Read the model definition and answer for the solid it produces. Units are mm, in the model's axes. A direction names the side the tool comes from. Coordinates: 2 decimals unless noted, no trailing zeros. Order: outer loops, then holes, each group sorted by start corner. A loop starts at its lowest first (then second) coordinate and runs counter-clockwise, first axis right, second up. Notation, with made-up numbers: M 77,63.5 L 102,63.5 A17 cw 102,90.5 Z; hole C -24.5,-29.75 d7. An arc over 180 degrees is marked long. One line per question, with ' | ' between items. Start each with the question number.
1) Find section B-B, the plane z = 44.5. Write down the section's boundary in (x, y).
2) The mould has two halves that part along X. Classify faces 3 (the face through (-25, -1, 75)), 4 (the face through (-23.66, -0.67, 73.51)), 5 (the face through (-1, 50, 38)): +X half, -X half, draft (parallel to the pull), parting line (faces both ways), or undercut.
3) Consider probe 1 along Y at (x, z) = (-19, 58); probe 2 along Y at (x, z) = (-9, 16.5). Determine where each line is inside the solid, lowest interval first.
4) A tool of negligible diameter and unlimited length cuts with its end or side. For faces 1 (the face through (-1, -48, 48)), 2 (the face through (36.15, 0.36, 62.41)), from which of +Z, -Z, +X, -X, +Y, -Y can it reach the whole face along a straight path? Write none if from no direction.
5) Find section D-D, the plane z = 19. Write down the section's boundary in (x, y), plus the area to 3 significant figures.
6) Given P1, Ø1, axis at x = -2.5, y = -49.5, coming from the -Z side; P2, Ø10, axis at y = 39, z = 77.5, coming from the -X side; P3, Ø5, axis at x = 13.5, y = 39.5, coming from the -Z side, each flat-ended and moving along its own axis, determine where each tip first touches the part or whether it passes through.
from build123d import *

# Parameters (mm, degrees)
F0_W     = 100
F0_H     = 100
F1_DEPTH = 100
F2_SIZE2 = 49.99999
F2_SIZE  = 49.99999
F3_T     = -2
F4_W     = 23.5146284103
F4_H     = 39.5418182015
F5_DEPTH = 2
F7_D     = 12.6
F7_DEPTH = 17.25
F7_TIP   = 3.7854218999


# Not quite as in the source:
# - a fillet or chamfer is up to 0.001 mm smaller than in the source, because OpenCascade refuses the exact size


with BuildPart() as f1:
    # F0 (on Top) → F1 (new body)
    with BuildSketch(Plane.XY):
        Rectangle(F0_W, F0_H)
    extrude(amount=F1_DEPTH)

    # F2 (size 50 and 50 in the source; OpenCascade refuses exactly that, so slightly less here)
    f2_edges = [f1.edges().sort_by_distance(p)[0] for p in [
        (-50, 0, 100),
        (50, 0, 100),
    ]]
    chamfer(f2_edges, length=F2_SIZE, length2=F2_SIZE2)

    # F3
    f3_openings = [f1.faces().sort_by_distance(p)[0] for p in [
        (0, 0, 0),
    ]]
    offset(amount=F3_T, openings=f3_openings)

    # F4 (on face) → F5 (cut, through all)
    with BuildSketch(Plane.XZ.offset(50)):
        with Locations((-0.3359224647, 19.7709091008)):
            Rectangle(F4_W, F4_H)
    extrude(amount=-F5_DEPTH, mode=Mode.SUBTRACT)

    # F7
    with Locations(Plane(origin=(50, 0, 50), x_dir=(0, 1, 0), z_dir=(0.7071067812, 0, 0.7071067812))):
        with Locations((17.1098317951, 50.0659272075), (-10.7799200341, 50.0659272075), (-23.6778985709, 30.9631545097), (3.2679832075, 24.1581760347), (26.1959340423, 37.8756783903)):
            Hole(F7_D / 2, depth=F7_DEPTH)
            with Locations((0, 0, -(F7_DEPTH + F7_TIP / 2))):  # 118° drill point
                Cone(0, F7_D / 2, F7_TIP, mode=Mode.SUBTRACT)


solid = f1.part
Report:
1) outline: M -50,-50 L 50,-50 L 50,50 L -50,50 Z; hole M -48,-48 L 48,-48 L 48,48 L -48,48 Z
2) face 3: -X half | face 4: undercut | face 5: draft
3) probe 1: y = -50 to -48, 48 to 50 | probe 2: y = 48 to 50
4) face 1: -Z | face 2: none
5) outline: M -50,-50 L -12.09,-50 L -12.09,-48 L -48,-48 L -48,48 L 48,48 L 48,-48 L 11.42,-48 L 11.42,-50 L 50,-50 L 50,50 L -50,50 Z | area: 737 mm^2
6) P1: stops at z = 39.54 | P2: stops at x = -27.5 | P3: stops at z = 81.17
